Model file for the job. Use its own axes, mm. A direction names the side the tool comes from. Round coordinates to 2 decimals unless told otherwise and drop trailing zeros. Order: outer loops, then holes, each group sorted by start corner. A loop starts at its lowest first (then second) coordinate and runs counter-clockwise, first axis right, second up. Notation, with made-up numbers: (-34, 12.5) -> (-1, 12.5) arc R25 cw to (-1, 40.5) -> close; hole circle Ø6 at (6.5, 74.5). An arc over 180 degrees is marked (long way). Use CSV: the item, a comma, the result in double quotes.
```python
from build123d import *

# Parameters (mm, degrees)
SKETCH_3_R          = 13
EXTRUDE_1_DEPTH     = 7.5
SKETCH_4_R          = 1.75
CUT_EXTRUDE_1_DEPTH = 8.5
SKETCH_5_R          = 2.8
CUT_EXTRUDE_2_DEPTH = 2.6
SKETCH_6_R          = 6
CUT_EXTRUDE_3_DEPTH = 8.5
SKETCH_7_R          = 13
SKETCH_7_R_2        = 2.8
EXTRUDE_2_DEPTH     = 3
CUT_EXTRUDE_4_DEPTH = 4
SKETCH_8_R          = 6
SKETCH_8_R_2        = 1.85
EXTRUDE_3_DEPTH     = 5


with BuildPart() as part:
    # ｽｹｯﾁ3 → ﾎﾞｽ - 押し出し1 (new body)
    with BuildSketch(Plane.XY):
        Circle(SKETCH_3_R)
    extrude(amount=EXTRUDE_1_DEPTH)

    # ｽｹｯﾁ4 → ｶｯﾄ - 押し出し1 (cut, through all)
    with BuildSketch(Plane.XY.offset(7.5)):
        with Locations((0, 10)):
            Circle(SKETCH_4_R)
        with Locations((8.660254038, -5)):
            Circle(SKETCH_4_R)
        with Locations((-8.660254038, -5)):
            Circle(SKETCH_4_R)
    extrude(amount=-CUT_EXTRUDE_1_DEPTH, mode=Mode.SUBTRACT)

    # ｽｹｯﾁ5 → ｶｯﾄ - 押し出し2 (cut)
    with BuildSketch(Plane(origin=(0, 0, 0), x_dir=(-1, 0, 0), z_dir=(0, 0, -1))):
        with Locations((8.660254038, -5)):
            Circle(SKETCH_5_R)
        with Locations((0, 10)):
            Circle(SKETCH_5_R)
        with Locations((-8.660254038, -5)):
            Circle(SKETCH_5_R)
    extrude(amount=-CUT_EXTRUDE_2_DEPTH, mode=Mode.SUBTRACT)

    # ｽｹｯﾁ6 → ｶｯﾄ - 押し出し3 (cut, through all)
    with BuildSketch(Plane.XY.offset(7.5)):
        Circle(SKETCH_6_R)
    extrude(amount=-CUT_EXTRUDE_3_DEPTH, mode=Mode.SUBTRACT)

    # ｽｹｯﾁ7 → ﾎﾞｽ - 押し出し2 (add)
    with BuildSketch(Plane(origin=(0, 0, 0), x_dir=(-1, 0, 0), z_dir=(0, 0, -1))):
        Circle(SKETCH_7_R)
        with Locations((0, 10)):
            Circle(SKETCH_7_R_2, mode=Mode.SUBTRACT)
        with Locations((8.660254038, -5)):
            Circle(SKETCH_7_R_2, mode=Mode.SUBTRACT)
        with Locations((-8.660254038, -5)):
            Circle(SKETCH_7_R_2, mode=Mode.SUBTRACT)
    extrude(amount=EXTRUDE_2_DEPTH)

    # ｽｹｯﾁ2 → ｶｯﾄ - 押し出し4 (cut, through all)
    with BuildSketch(Plane.XY):
        with BuildLine():
            Line((-3.75, 6.495190528), (-2.463350586, 13.926501921))
            ThreePointArc((-2.463350586, 13.926501921), (0, 16), (2.463350586, 13.926501921))
            Line((2.463350586, 13.926501921), (3.75, 6.495190528))
            Line((3.75, 6.495190528), (10.829029157, 9.096575147))
            ThreePointArc((10.829029157, 9.096575147), (13.856406461, 8), (13.292379743, 4.829926775))
            Line((13.292379743, 4.829926775), (7.5, 0))
            Line((7.5, 0), (13.292379743, -4.829926775))
            ThreePointArc((13.292379743, -4.829926775), (13.856406461, -8), (10.829029157, -9.096575147))
            Line((10.829029157, -9.096575147), (3.75, -6.495190528))
            Line((3.75, -6.495190528), (2.463350586, -13.926501921))
            ThreePointArc((2.463350586, -13.926501921), (0, -16), (-2.463350586, -13.926501921))
            Line((-2.463350586, -13.926501921), (-3.75, -6.495190528))
            Line((-3.75, -6.495190528), (-10.829029157, -9.096575147))
            ThreePointArc((-10.829029157, -9.096575147), (-13.856406461, -8), (-13.292379743, -4.829926775))
            Line((-13.292379743, -4.829926775), (-7.5, 0))
            Line((-7.5, 0), (-13.292379743, 4.829926775))
            ThreePointArc((-13.292379743, 4.829926775), (-13.856406461, 8), (-10.829029157, 9.096575147))
            Line((-10.829029157, 9.096575147), (-3.75, 6.495190528))
        make_face()
    extrude(amount=-CUT_EXTRUDE_4_DEPTH, mode=Mode.SUBTRACT)

    # ｽｹｯﾁ8 → ﾎﾞｽ - 押し出し3 (add)
    with BuildSketch(Plane(origin=(0, 0, 0), x_dir=(-1, 0, 0), z_dir=(0, 0, -1))):
        Circle(SKETCH_8_R)
        Circle(SKETCH_8_R_2, mode=Mode.SUBTRACT)
    extrude(amount=-EXTRUDE_3_DEPTH)


solid = part.part
```
Q1. Cut at A-A (z = -1.25). Give the cut face in (x, y), plus the area to 3 significant figures.
From the geometry:
outline,"(-12.35, -4.05) -> (-7.5, 0) -> (-12.35, 4.05) arc R13 ccw to start; (-9.68, -8.68) arc R13 ccw to (-2.67, -12.72) -> (-3.75, -6.5) -> close; (-9.68, 8.68) -> (-3.75, 6.5) -> (-2.67, 12.72) arc R13 ccw to start; (2.67, -12.72) arc R13 ccw to (9.68, -8.68) -> (3.75, -6.5) -> close; (2.67, 12.72) -> (3.75, 6.5) -> (9.68, 8.68) arc R13 ccw to start; (7.5, 0) -> (12.35, -4.05) arc R13 ccw to (12.35, 4.05) -> close"
area,"139 mm²"
Q2. Which spindle directions (+Z, -Z, +X, -X, +Y, -Y) get a long thin tool onto all of the face, cutting with end or side? Do faces 1 (the cylindrical face through (-6, 0, 6)), 2 (the flat face through (5, 10, -3)), 3 (the flat face through (9.9, -2, -1.5)), 4 (the flat face through (-6.67, -7.57, -1.48)). Say none if no direction does.
From the geometry:
face 1,"+Z"
face 2,"-Z, +X, -X, +Y, -Y"
face 3,"-Z"
face 4,"-Z, -X"
Q3. Probe line 1 along Y through (x, z) = (0, 1.35); line 2 along Y through (x, z) = (0, 6.15); line 3 along Z through (x, y) = (10, 5.75). List the from-to ranges inside material, lowest first.
From the geometry:
line 1,"y = -13 to -1.85, 1.85 to 7.2, 12.8 to 13"
line 2,"y = -13 to -6, 6 to 8.25, 11.75 to 13"
line 3,"z = 0 to 7.5"
Q4. Cut at C-C (z = 4). Give the cut face in (x, y).
From the geometry:
outline,"circle Ø26 at (0, 0); hole circle Ø3.5 at (-8.66, -5); hole circle Ø3.7 at (0, 0); hole circle Ø3.5 at (0, 10); hole circle Ø3.5 at (8.66, -5)"
Q5. Pin check, flat tips, straight feed: pin 1 (5 mm diameter, centred on x = 6, z = 3, fed in from -Y); pin 2 (4.5 mm diameter, centred on x = 9.5, y = -6, fed in from -Z); pin 3 (6 mm diameter, centred on x = -5, z = -1, fed in from -Y); pin 4 (3 mm diameter, centred on x = 1, z = 2, fed in from +Y). Stop position of each tip, or through.
From the geometry:
pin 1,"stops at y = -12.52"
pin 2,"stops at z = 0"
pin 3,"stops at y = -12.82"
pin 4,"stops at y = 13"
Q6. Cut at D-D (y = -4.5). Give the cut face in (x, z), plus the area to 3 significant figures.
From the geometry:
outline,"(-12.2, 0) -> (-11.42, 0) -> (-11.42, 2.6) -> (-10.34, 2.6) -> (-10.34, 7.5) -> (-12.2, 7.5) -> close; (-6.98, 2.6) -> (-5.91, 2.6) -> (-5.91, 0) -> (5.91, 0) -> (5.91, 2.6) -> (6.98, 2.6) -> (6.98, 7.5) -> (3.97, 7.5) -> (3.97, 5) -> (-3.97, 5) -> (-3.97, 7.5) -> (-6.98, 7.5) -> close; (10.34, 2.6) -> (11.42, 2.6) -> (11.42, 0) -> (12.2, 0) -> (12.2, 7.5) -> (10.34, 7.5) -> close"
area,"102 mm²"
Q7. Mould opens along X. For faces 5 (the flat face through (6.67, 7.57, -1.48)), 6 (the flat face through (1.42, 1.42, 5)), 7 (the flat face through (3, -6, 7.5)), 8 (the flat face through (3.203, 9.652, -1.479)) say: +X half, -X half, draft (parallel to the pull), parting line (faces both ways), or undercut.
From the geometry:
face 5,"+X half"
face 6,"undercut"
face 7,"draft"
face 8,"undercut"
